Design review of the part built by this model. Coordinates are the model's own, in mm. Face numbers are marked on the shaded views. A direction names the side the tool comes from. Give positions to 0.01 mm unless a question says otherwise; leave off trailing zeros. Write each loop counter-clockwise with the first axis right and the second up, starting at its lowest first coordinate (ties: lowest second). Pieces come first, ordered by that corner, then holes. Notation, with made-up numbers: (25, -39.5) -> (54, -39.5) arc R19 ccw to (54, -13.5) -> close; hole circle Ø9 at (-26, 80.25). An arc over 180 degrees is marked (long way). Answer as a JSON object with one key per item and string values.
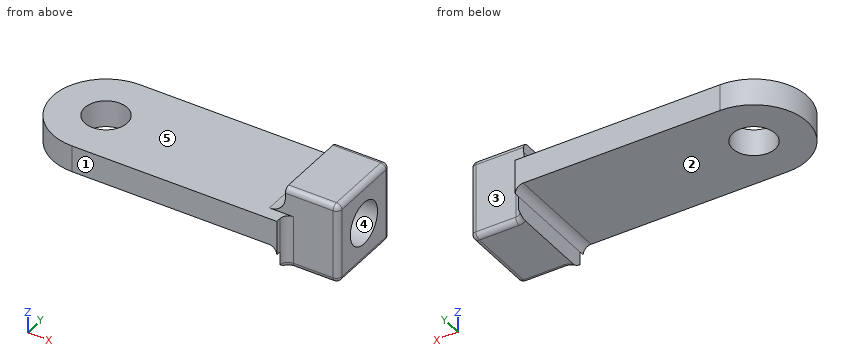
```python
from build123d import *

# Parameters (mm, degrees)
SKETCH1_R           = 4
BOSS_EXTRUDE1_DEPTH = 5
SKETCH2_W           = 25.16319253
SKETCH2_H           = 20
CUT_EXTRUDE1_DEPTH  = 35.369317712
SKETCH3_W           = 15
SKETCH3_H           = 15
BOSS_EXTRUDE2_DEPTH = 10
FILLET1_R           = 1.5
FILLET2_R           = 3
SKETCH4_R           = 4
CUT_EXTRUDE2_DEPTH  = 8
FILLET3_R           = 1
FILLET4_R           = 1


with BuildPart() as part:
    # Sketch1 → Boss-Extrude1 (new body)
    with BuildSketch(Plane.XY):
        with BuildLine():
            Line((-22.5, 10), (22.5, 10))
            ThreePointArc((22.5, 10), (32.5, 0), (22.5, -10))
            Line((22.5, -10), (-22.5, -10))
            ThreePointArc((-22.5, -10), (-32.5, 0), (-22.5, 10))
        make_face()
        with Locations((-22.5, 0)):
            Circle(SKETCH1_R, mode=Mode.SUBTRACT)
        with Locations((22.5, 0)):
            Circle(SKETCH1_R, mode=Mode.SUBTRACT)
    extrude(amount=BOSS_EXTRUDE1_DEPTH)

    # Sketch2 → Cut-Extrude1 (cut, through all)
    with BuildSketch(Plane.XY.offset(5)):
        with Locations((28.623168012, 0)):
            Rectangle(SKETCH2_W, SKETCH2_H)
    extrude(amount=-CUT_EXTRUDE1_DEPTH, mode=Mode.SUBTRACT)

    # Sketch3 → Boss-Extrude2 (add)
    with BuildSketch(Plane(origin=(16.041571747, 0, 0), x_dir=(0, 0, -1), z_dir=(1, 0, 0))):
        with Locations((-2.5, 0)):
            Rectangle(SKETCH3_W, SKETCH3_H)
    extrude(amount=BOSS_EXTRUDE2_DEPTH)

    # Fillet1
    # the kernel refuses this fillet: 1.5 mm, written as the material it adds along each edge
    with BuildSketch(Plane(origin=(16.041571747, 11.25, 0), x_dir=(-1, 0, 0), z_dir=(0, -1, 0))) as fillet1_piece_1_section:
        with BuildLine():
            CenterArc((FILLET1_R, FILLET1_R), FILLET1_R, 180, 90)
            Line((0, FILLET1_R), (0, 0))
            Line((0, 0), (FILLET1_R, 0))
        make_face()
    fillet1_piece_1 = extrude(amount=22.5, mode=Mode.PRIVATE)
    fillet1_piece_1 = split(fillet1_piece_1, bisect_by=Plane(origin=(16.041571747, 10, 0), z_dir=(0, -1, 0)), keep=Keep.TOP, mode=Mode.PRIVATE)
    fillet1_piece_1 = split(fillet1_piece_1, bisect_by=Plane(origin=(16.041571747, -10, 0), z_dir=(0, 1, 0)), keep=Keep.TOP, mode=Mode.PRIVATE)
    add(fillet1_piece_1)
    # the kernel refuses this fillet: 1.5 mm, written as the material it adds along each edge
    with BuildSketch(Plane(origin=(16.041571747, 7.5, 5), x_dir=(1, 0, 0), z_dir=(0, 0, -1))) as fillet1_2_piece_1_section:
        with BuildLine():
            CenterArc((FILLET1_R, -FILLET1_R), FILLET1_R, 90, 90)
            Line((0, -FILLET1_R), (0, 0))
            Line((0, 0), (FILLET1_R, 0))
        make_face()
    fillet1_2_piece_1 = extrude(amount=10.25, mode=Mode.PRIVATE)
    fillet1_2_piece_1 = split(fillet1_2_piece_1, bisect_by=Plane(origin=(16.041571747, 7.5, -5), z_dir=(0, 0, 1)), keep=Keep.TOP, mode=Mode.PRIVATE)
    add(fillet1_2_piece_1)
    # the kernel refuses this fillet: 1.5 mm, written as the material it adds along each edge
    with BuildSketch(Plane(origin=(16.041571747, -7.5, -5.25), x_dir=(1, 0, 0), z_dir=(0, 0, 1))) as fillet1_3_piece_1_section:
        with BuildLine():
            CenterArc((FILLET1_R, -FILLET1_R), FILLET1_R, 90, 90)
            Line((0, -FILLET1_R), (0, 0))
            Line((0, 0), (FILLET1_R, 0))
        make_face()
    fillet1_3_piece_1 = extrude(amount=10.25, mode=Mode.PRIVATE)
    fillet1_3_piece_1 = split(fillet1_3_piece_1, bisect_by=Plane(origin=(16.041571747, -7.5, -5), z_dir=(0, 0, 1)), keep=Keep.TOP, mode=Mode.PRIVATE)
    add(fillet1_3_piece_1)

    # Fillet2
    fillet2_edges = [part.edges().sort_by_distance(p)[0] for p in [
        (16.041571747, 0, 5),
    ]]
    fillet(fillet2_edges, radius=FILLET2_R)

    # Sketch4 → Cut-Extrude2 (cut)
    with BuildSketch(Plane(origin=(26.041571747, 0, 0), x_dir=(0, 0, -1), z_dir=(1, 0, 0))):
        with Locations((-2.5, 0)):
            Circle(SKETCH4_R)
    extrude(amount=-CUT_EXTRUDE2_DEPTH, mode=Mode.SUBTRACT)

    # Fillet3
    fillet3_edges = [part.edges().sort_by_distance(p)[0] for p in [
        (21.791571747, -7.5, -5),
        (21.791571747, 7.5, -5),
        (21.041571747, 7.5, 10),
        (21.041571747, -7.5, 10),
        (16.480911575, 7.939339828, -5),
        (16.480911575, -7.939339828, -5),
    ]]
    fillet(fillet3_edges, radius=FILLET3_R)

    # Fillet4
    fillet4_edges = [part.edges().sort_by_distance(p)[0] for p in [
        (26.041571747, 0, -5),
        (26.041571747, -7.5, 2.5),
        (26.041571747, 7.5, 2.5),
        (26.041571747, 0, 10),
        (26.041571747, 7.207106781, -4.707106781),
        (26.041571747, 7.207106781, 9.707106781),
        (26.041571747, -7.207106781, 9.707106781),
        (26.041571747, -7.207106781, -4.707106781),
    ]]
    fillet(fillet4_edges, radius=FILLET4_R)


solid = part.part
```
(1) We need section C-C, the plane y = -5.25. State the section outline as (x, z) points, then the cut area to 3 significant figures.
Here are the results:
{"outline": "(-31.01, 0) -> (14.54, 0) arc R1.5 cw to (16.04, -1.5) -> (16.04, -5) -> (25.04, -5) arc R1 ccw to (26.04, -4) -> (26.04, 9) arc R1 ccw to (25.04, 10) -> (16.04, 10) -> (16.04, 8) arc R3 cw to (13.04, 5) -> (-31.01, 5) -> close", "area": "387 mm²"}
(2) We need section B-B, the plane y = 0. State the section outline as (x, z) points.
Here are the results:
{"outline": "(-32.5, 0) -> (-26.5, 0) -> (-26.5, 5) -> (-32.5, 5) -> close; (-18.5, 0) -> (14.54, 0) arc R1.5 cw to (16.04, -1.5) -> (16.04, -5) -> (25.04, -5) arc R1 ccw to (26.04, -4) -> (26.04, -1.5) -> (18.04, -1.5) -> (18.04, 6.5) -> (26.04, 6.5) -> (26.04, 9) arc R1 ccw to (25.04, 10) -> (16.04, 10) -> (16.04, 8) arc R3 cw to (13.04, 5) -> (-18.5, 5) -> close"}
(3) For line 1 along Y through (x, z) = (-22.5, 2.95); line 2 along Z through (x, y) = (-27, 3.75); line 3 along Y through (x, z) = (24.25, 2.5), list the stretches that pass through material, from the lowest coordinate up.
Here are the results:
{"line 1": "y = -10 to -4, 4 to 10", "line 2": "z = 0 to 5", "line 3": "y = -7.5 to -4, 4 to 7.5"}
(4) The part is to be moulded in two halves that separate along Z. For the marked faces 3, 4 and 5, say which applies: +Z half, -Z half, draft (parallel to the pull), parting line (faces both ways), or undercut.
Here are the results:
{"face 3": "draft", "face 4": "undercut", "face 5": "+Z half"}
(5) Clearance check with flat-ended pins moving along their axes: pin 1 (4 mm diameter, centred on y = -0.5, z = -3.5, fed in from -X); pin 2 (1.1 mm diameter, centred on y = 9.5, z = 0.5, fed in from +X); pin 3 (1.5 mm diameter, centred on x = 15.5, z = 7.5, fed in from -Y). State where each tip first meets the part, or that it passes through.
Here are the results:
{"pin 1": "stops at x = 16.04", "pin 2": "stops at x = 16.04", "pin 3": "stops at y = -7.5"}
(6) We need section D-D, the plane x = -6. State the section outline as (y, z) points, then the cut area to 3 significant figures.
Here are the results:
{"outline": "(-10, 0) -> (10, 0) -> (10, 5) -> (-10, 5) -> close", "area": "100 mm²"}
(7) For the marked faces 1 and 2, list the 3-axis set-ups (+Z, -Z, +X, -X, +Y, -Y) from which the entire face can be reached by the end or side of a thin tool; tool diameter is ignored.
Here are the results:
{"face 1": "+Z, -Z, +X, -X, -Y", "face 2": "-Z, -X, +Y, -Y"}
(8) We need section A-A, the plane z = 2.5. State the section outline as (x, y) points.
Here are the results:
{"outline": "(-22.5, -10) -> (16.04, -10) -> (16.04, -9) arc R1.5 cw to (17.54, -7.5) -> (25.04, -7.5) arc R1 ccw to (26.04, -6.5) -> (26.04, -4) -> (18.04, -4) -> (18.04, 4) -> (26.04, 4) -> (26.04, 6.5) arc R1 ccw to (25.04, 7.5) -> (17.54, 7.5) arc R1.5 cw to (16.04, 9) -> (16.04, 10) -> (-22.5, 10) arc R10 ccw to start; hole circle Ø8 at (-22.5, 0)"}
